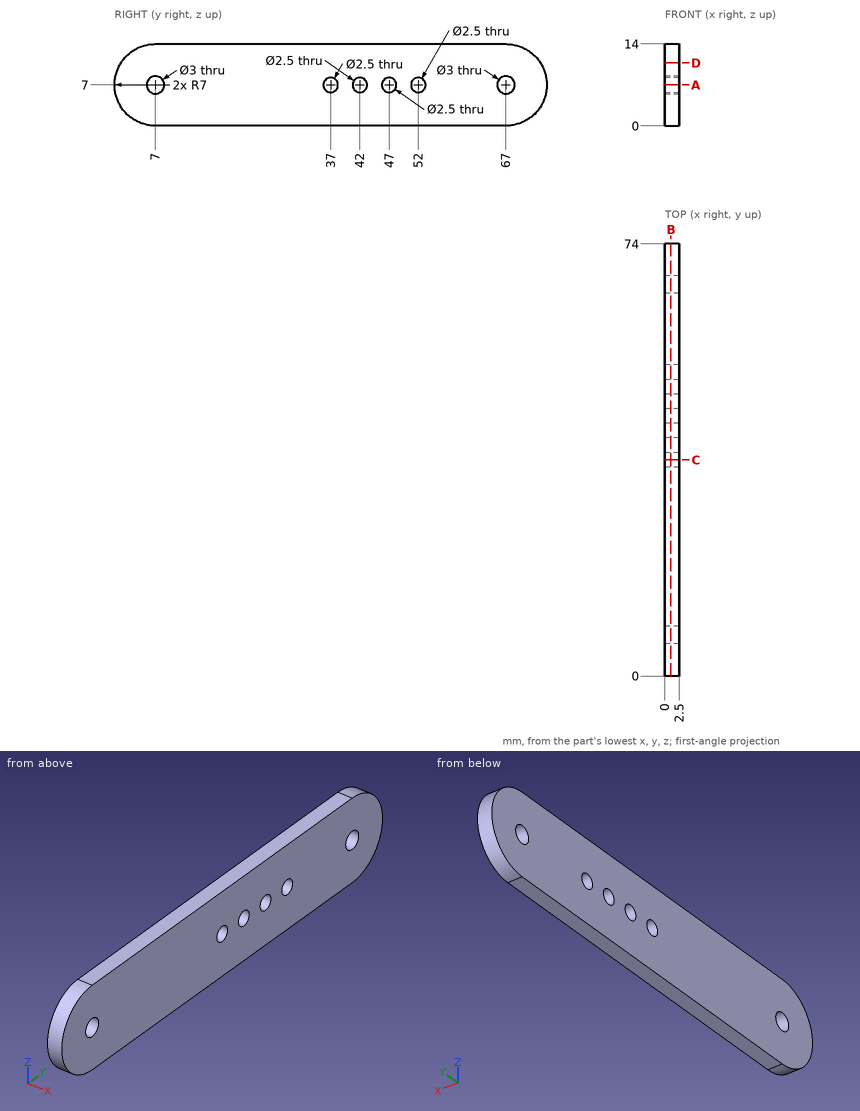
Part print with two shaded views. Sizes in mm from the minimum x, y, z corner. Coordinates: 2 decimals unless noted, no trailing zeros. Order: outer loops, then holes, each group sorted by start corner. A loop starts at its lowest first (then second) coordinate and runs counter-clockwise, first axis right, second up. Notation, with made-up numbers: M 75.25,74 L 134.25,74 A22 ccw 134.25,108 Z; hole C 57,27.5 d1. An arc over 180 degrees is marked long. One line per question, with ' | ' between items. Start each with the question number.
1. Cut at C-C (y = 37). Write the cut outline in (x, z).
2. Cut at A-A (z = 7). Write the cut outline in (x, y), plus the area to 3 significant figures.
3. Flat gauge pins, fed straight in: P1, Ø1.5, axis at x = 2, z = 8, coming from the +Y side; P2, Ø2, axis at y = 37, z = 7, coming from the -X side. Where does each tip first touch, or does it go through?
4. Cut at B-B (x = 1.05). Write the cut outline in (y, z).
5. Cut at D-D (z = 10.75). Write the cut outline in (x, y).
6. Wall check: line 1 along Z through (x, y) = (1.05, 43); line 2 along Z through (x, y) = (1.2, 37.5); line 3 along Y through (x, z) = (1.45, 1.25). Give the ranges that are in metal, low to high. Write a range as [from, to].
The answers:
1) outline: M 0,0 L 2.5,0 L 2.5,5.75 L 0,5.75 Z; M 0,8.25 L 2.5,8.25 L 2.5,14 L 0,14 Z
2) outline: M 0,0 L 2.5,0 L 2.5,5.5 L 0,5.5 Z; M 0,8.5 L 2.5,8.5 L 2.5,35.75 L 0,35.75 Z; M 0,38.25 L 2.5,38.25 L 2.5,40.75 L 0,40.75 Z; M 0,43.25 L 2.5,43.25 L 2.5,45.75 L 0,45.75 Z; M 0,48.25 L 2.5,48.25 L 2.5,50.75 L 0,50.75 Z; M 0,53.25 L 2.5,53.25 L 2.5,65.5 L 0,65.5 Z; M 0,68.5 L 2.5,68.5 L 2.5,74 L 0,74 Z | area: 145 mm2
3) P1: stops at y = 74 | P2: passes through
4) outline: M 7,0 L 67,0 A7 ccw 67,14 L 7,14 A7 ccw Z; hole C 7,7 d3; hole C 37,7 d2.5; hole C 42,7 d2.5; hole C 47,7 d2.5; hole C 52,7 d2.5; hole C 67,7 d3
5) outline: M 0,1.09 L 2.5,1.09 L 2.5,72.91 L 0,72.91 Z
6) line 1: z = [0, 6.25], [7.75, 14] | line 2: z = [0, 5.85], [8.15, 14] | line 3: y = [3.01, 70.99]
